Geometry check sheet. Reference: the model listing, model coordinates, mm. Face numbers are marked on the shaded views. A direction names the side the tool comes from. Round coordinates to 2 decimals unless told otherwise and drop trailing zeros. Write each loop counter-clockwise with the first axis right and the second up, starting at its lowest first coordinate (ties: lowest second). Pieces come first, ordered by that corner, then holes. Notation, with made-up numbers: (18.25, 47) -> (27.25, 47) arc R16 cw to (27.25, 55) -> close; hole circle Ø4 at (-4.5, -12). An arc over 180 degrees is marked (long way). Return JSON: item names as keys, results as strings. Group by question number.
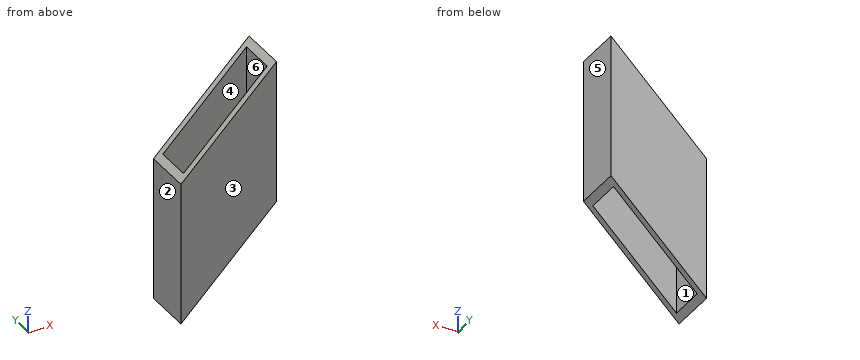
from build123d import *

# Parameters (mm, degrees)
SKETCH1_W           = 50.8
SKETCH1_H           = 25.4
SKETCH1_W_2         = 44.45
SKETCH1_H_2         = 19.05
BOSS_EXTRUDE1_DEPTH = 127
CUT_EXTRUDE1_DEPTH  = 127


with BuildPart() as part:
    # Sketch1 → Boss-Extrude1 (new body)
    with BuildSketch(Plane.XY):
        with Locations((25.4, 12.7)):
            Rectangle(SKETCH1_W, SKETCH1_H)
        with Locations((25.4, 12.7)):
            Rectangle(SKETCH1_W_2, SKETCH1_H_2, mode=Mode.SUBTRACT)
    extrude(amount=BOSS_EXTRUDE1_DEPTH)

    # Sketch2 → Cut-Extrude1 (cut)
    with BuildSketch(Plane(origin=(0, 25.4, 0), x_dir=(1, 0, 0), z_dir=(0, 1, 0))):
        Polygon((0, 0), (50.8, -50.8), (50.8, 0), align=None)
        Polygon((0, -76.2), (0, -127), (50.8, -127), align=None)
    extrude(amount=-CUT_EXTRUDE1_DEPTH, mode=Mode.SUBTRACT)


solid = part.part
1) Sectioned sample at A-A on y = 20.5. Enter the section's corners in (x, z) (3 decimals), and give its area (3 significant figures).
2) Go/stop test with flat-tipped pins: P1, Ø5.5, axis at y = 11.5, z = 102, coming from the -X side (3 decimals); P2, Ø1, axis at y = 21, z = 38.5, coming from the +X side (3 decimals); P3, Ø4, axis at x = 27.5, y = 7, coming from the +Z side. Record where each tip stops, or that it passes through.
3) Sectioned sample at D-D on z = 65.5. Enter the section's corners in (x, y) (3 decimals).
4) Tool access check on the marked faces 1 and 2. Record the directions out of +Z, -Z, +X, -X, +Y, -Y that give a thin tool (end or side, any length) a straight path to the whole face; none if there is none.
5) Sectioned sample at B-B on z = 102.5. Enter the section's corners in (x, y) (3 decimals), and give its area (3 significant figures).
6) Sectioned sample at C-C on x = 29.5. Enter the section's corners in (y, z) (3 decimals), and give its area (3 significant figures).
7) Mould release check, pull along X, two halves, no side actions. Record for the marked faces 3, 4, 5 and 6: +X half, -X half, draft (parallel to the pull), parting line (faces both ways), or undercut.
8) Material ranges on probe 1 along Y at (x, z) = (40, 54) (3 decimals); probe 2 along X at (y, z) = (21.5, 66) (3 decimals); probe 3 along X at (y, z) = (6.75, 117) (3 decimals), recorded low to high. Write a range as [from, to].
Evaluation:
{
 "1": {"outline": "(0, 0) -> (3.175, 3.175) -> (3.175, 79.375) -> (0, 76.2) -> close; (47.625, 47.625) -> (50.8, 50.8) -> (50.8, 127) -> (47.625, 123.825) -> close", "area": "484 mm2"},
 "2": {"P1": "stops at x = 47.625", "P2": "stops at x = 3.175", "P3": "passes through"},
 "3": {"outline": "(0, 0) -> (50.8, 0) -> (50.8, 25.4) -> (0, 25.4) -> close; hole (3.175, 3.175) -> (47.625, 3.175) -> (47.625, 22.225) -> (3.175, 22.225) -> close"},
 "4": {"face 1": "+Z, -Z", "face 2": "+Z, -Z, -X, +Y, -Y"},
 "5": {"outline": "(26.3, 0) -> (50.8, 0) -> (50.8, 25.4) -> (26.3, 25.4) -> (26.3, 22.225) -> (47.625, 22.225) -> (47.625, 3.175) -> (26.3, 3.175) -> close", "area": "216 mm2"},
 "6": {"outline": "(0, 29.5) -> (3.175, 29.5) -> (3.175, 105.7) -> (0, 105.7) -> close; (22.225, 29.5) -> (25.4, 29.5) -> (25.4, 105.7) -> (22.225, 105.7) -> close", "area": "484 mm2"},
 "7": {"face 3": "draft", "face 4": "undercut", "face 5": "+X half", "face 6": "undercut"},
 "8": {"probe 1": "y = [0, 3.175], [22.225, 25.4]", "probe 2": "x = [0, 3.175], [47.625, 50.8]", "probe 3": "x = [47.625, 50.8]"}
}
